Design review of the part built by this model. Coordinates are the model's own, in mm. Give positions to 0.01 mm unless a question says otherwise; leave off trailing zeros. Order: outer loops, then holes, each group sorted by start corner. A loop starts at its lowest first (then second) coordinate and runs counter-clockwise, first axis right, second up. Notation, with made-up numbers: (35.25, 57) -> (39.25, 57) arc R25 ccw to (39.25, 89) -> close; hole circle Ø9 at (-7, 6). An arc over 180 degrees is marked (long way). One line per item, written item: value. Start each with the question number.
1) Consider section C-C (x = 26.5). State the section outline as (y, z) points, plus the area to 3 significant figures.
2) Wall thickness on line 1 along X through (y, z) = (11.5, 0.85); line 2 along X through (y, z) = (33, 3.5); line 3 along Y through (x, z) = (4, 2.9): over which ranges is each line inside the solid? List them lowest first. Write a range as from..to.
3) The part is to be moulded in two halves that separate along Y. For faces 1 (the face through (0, 41, 4)), 2 (the face through (39.328, -22.766, 1.972)), 3 (the face through (21.51, -37.81, 1.97)), say which applies: released by +Y, released by -Y, zero draft, split by the parting line, or undercut.
4) For pin 1 (2 mm diameter, centred on x = 22.5, z = 3.5, fed in from -Y); pin 2 (1.5 mm diameter, centred on x = 7.5, z = 3.5, fed in from -Y), all flat-tipped, find the tip position at first contact; note any pin that passes through.
5) Consider section B-B (z = 2.2). State the section outline as (x, y) points, plus the area to 3 significant figures.
6) Consider section A-A (y = 0). State the section outline as (x, z) points, plus the area to 3 significant figures.
from build123d import *

# Parameters (mm, degrees)
F0_R     = 0.942302
F0_R_2   = 40.5
F1_DEPTH = 4


with BuildPart() as f1:
    # F0 (on Top) → F1 (new body)
    with BuildSketch(Plane.XY):
        with BuildLine():
            ThreePointArc((2.79807, 43.409916), (0, 45.442302), (-2.79807, 43.409916))
            ThreePointArc((-2.79807, 43.409916), (-21.75, 37.672105), (-36.195055, 24.128158))
            ThreePointArc((-36.195055, 24.128158), (-39.354188, 22.721151), (-38.993125, 19.281758))
            ThreePointArc((-38.993125, 19.281758), (-43.5, 0), (-38.993125, -19.281758))
            ThreePointArc((-38.993125, -19.281758), (-39.354188, -22.721151), (-36.195055, -24.128158))
            ThreePointArc((-36.195055, -24.128158), (-21.75, -37.672105), (-2.79807, -43.409916))
            ThreePointArc((-2.79807, -43.409916), (0, -45.442302), (2.79807, -43.409916))
            ThreePointArc((2.79807, -43.409916), (21.75, -37.672105), (36.195055, -24.128158))
            ThreePointArc((36.195055, -24.128158), (39.354188, -22.721151), (38.993125, -19.281758))
            ThreePointArc((38.993125, -19.281758), (43.5, 0), (38.993125, 19.281758))
            ThreePointArc((38.993125, 19.281758), (39.354188, 22.721151), (36.195055, 24.128158))
            ThreePointArc((36.195055, 24.128158), (21.75, 37.672105), (2.79807, 43.409916))
        make_face()
        with Locations((-36.80608, -21.25)):
            Circle(F0_R, mode=Mode.SUBTRACT)
        with Locations((0, -42.5)):
            Circle(F0_R, mode=Mode.SUBTRACT)
        with Locations((36.80608, -21.25)):
            Circle(F0_R, mode=Mode.SUBTRACT)
        with Locations((-36.80608, 21.25)):
            Circle(F0_R, mode=Mode.SUBTRACT)
        Circle(F0_R_2, mode=Mode.SUBTRACT)
        with Locations((36.80608, 21.25)):
            Circle(F0_R, mode=Mode.SUBTRACT)
        with Locations((0, 42.5)):
            Circle(F0_R, mode=Mode.SUBTRACT)
    extrude(amount=F1_DEPTH)


solid = f1.part
Checked values:
1. outline: (-34.5, 0) -> (-30.63, 0) -> (-30.63, 4) -> (-34.5, 4) -> close; (30.63, 0) -> (34.5, 0) -> (34.5, 4) -> (30.63, 4) -> close
1. area: 31.0 mm^2
2. line 1: x = -41.95..-38.83, 38.83..41.95
2. line 2: x = -28.34..-23.48, 23.48..28.34
2. line 3: y = -43.32..-40.3, 40.3..43.32
3. face 1: zero draft
3. face 2: undercut
3. face 3: released by -Y
4. pin 1: stops at y = -37.82
4. pin 2: stops at y = -42.97
5. outline: (-38.99, -19.28) arc R2.94 ccw to (-36.2, -24.13) arc R43.5 ccw to (-2.8, -43.41) arc R2.94 ccw to (2.8, -43.41) arc R43.5 ccw to (36.2, -24.13) arc R2.94 ccw to (38.99, -19.28) arc R43.5 ccw to (38.99, 19.28) arc R2.94 ccw to (36.2, 24.13) arc R43.5 ccw to (2.8, 43.41) arc R2.94 ccw to (-2.8, 43.41) arc R43.5 ccw to (-36.2, 24.13) arc R2.94 ccw to (-38.99, 19.28) arc R43.5 ccw to start; hole circle Ø81 at (0, 0); hole circle Ø1.88 at (-36.81, -21.25); hole circle Ø1.88 at (-36.81, 21.25); hole circle Ø1.88 at (0, -42.5); hole circle Ø1.88 at (0, 42.5); hole circle Ø1.88 at (36.81, -21.25); hole circle Ø1.88 at (36.81, 21.25)
5. area: 823 mm^2
6. outline: (-43.5, 0) -> (-40.5, 0) -> (-40.5, 4) -> (-43.5, 4) -> close; (40.5, 0) -> (43.5, 0) -> (43.5, 4) -> (40.5, 4) -> close
6. area: 24.0 mm^2
